Job drawing, mm, ordinate dimensions from the low corner. One solid piece. A direction names the side the tool comes from. Give positions to 0.01 mm unless a question says otherwise; leave off trailing zeros. Loops run counter-clockwise (first coordinate to the right, second up) from the corner with the lowest first, then second, coordinate; pieces in that order, holes last. Notation, with made-up numbers: M -37.5,29 L 8.5,29 A22 ccw 8.5,57 Z; hole C 40,16 d4. An arc over 180 degrees is marked long. Answer in a Markdown table with one row per item.
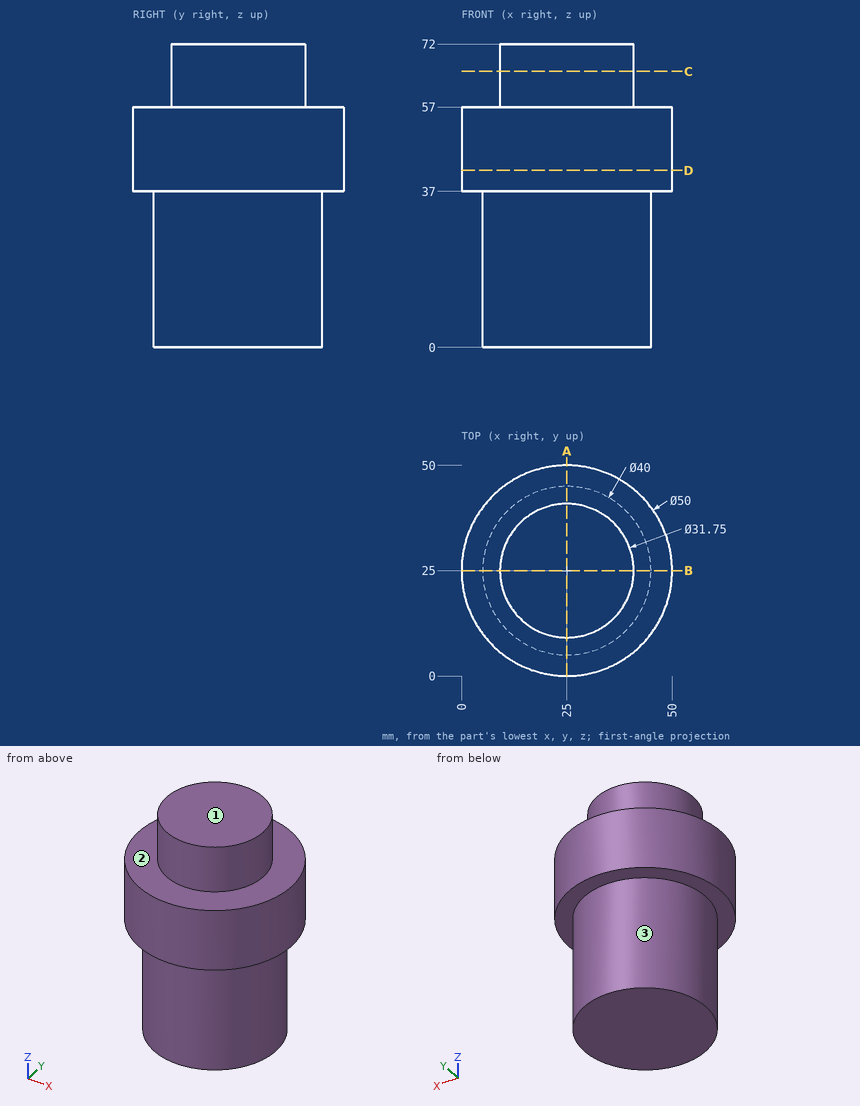
(1) Saw through at D-D (z = 42). Write the cut outline in (x, y), plus the area to 3 significant figures.
Recorded:
| item | result |
|---|---|
| outline | C 25,25 d50 |
| area | 1,960 mm^2 |
(2) Saw through at A-A (x = 25). Write the cut outline in (y, z) (3 decimals).
Recorded:
| item | result |
|---|---|
| outline | M 0,37 L 5,37 L 5,0 L 45,0 L 45,37 L 50,37 L 50,57 L 40.875,57 L 40.875,72 L 9.125,72 L 9.125,57 L 0,57 Z |
(3) Which spindle directions (+Z, -Z, +X, -X, +Y, -Y) get a long thin tool onto all of the face, cutting with end or side? Do the marked faces 1, 2 and 3. Say none if no direction does.
Recorded:
| item | result |
|---|---|
| face 1 | +Z, +X, -X, +Y, -Y |
| face 2 | +Z |
| face 3 | -Z |
(4) Saw through at C-C (z = 65.5). Write the cut outline in (x, y) (3 decimals), plus the area to 3 significant figures.
Recorded:
| item | result |
|---|---|
| outline | C 25,25 d31.75 |
| area | 792 mm^2 |
(5) Pin check, flat tips, straight feed: pin 1 Ø1.5 at (y, z) = (31, 24) entering from -X; pin 2 Ø12 at (x, y) = (8, 33.5) entering from +Z; pin 3 Ø5 at (x, z) = (8, 49.5) entering from -Y; pin 4 Ø6 at (x, y) = (18, 43) entering from +Z. Stop position of each tip, or through.
Recorded:
| item | result |
|---|---|
| pin 1 | stops at x = 5.7 |
| pin 2 | stops at z = 72 |
| pin 3 | stops at y = 4.63 |
| pin 4 | stops at z = 57 |
(6) Drill centre lines: line 1 along Z through (x, y) = (33, 40); line 2 along Z through (x, y) = (38.5, 9.5); line 3 along X through (y, z) = (40.5, 18.5). Where is each one in solid material? Low to high.
Recorded:
| item | result |
|---|---|
| line 1 | z = 0 to 57 |
| line 2 | z = 37 to 57 |
| line 3 | x = 12.36 to 37.64 |
